Part model, mm, in its own coordinate system. Face numbers are marked on the shaded views. A direction names the side the tool comes from. Round coordinates to 2 decimals unless told otherwise and drop trailing zeros. Loops run counter-clockwise (first coordinate to the right, second up) from the corner with the lowest first, then second, coordinate; pieces in that order, holes last.
1) Band-saw the part on C-C, the plane y = 0. Write the cut outline in (x, z), then the cut area to 4 significant figures.
2) Drop flat-ended pins along their axis: P1, Ø2, axis at x = 14, y = -2, coming from the -Z side; P2, Ø3, axis at y = 1, z = -26.5, coming from the -X side; P3, Ø5, axis at x = 11.5, y = 0, coming from the -Z side; P4, Ø6.5, axis at y = -5, z = -11, coming from the +X side. Give the stop position or say it passes through.
3) Band-saw the part on A-A, the plane y = -5. Write the cut outline in (x, z).
4) 3-axis set-ups, long thin cutter, end or side, ignore diameter. For the marked faces 1, 2, 3 and 4: which of +Z, -Z, +X, -X, +Y, -Y reach the whole face in a straight line?
5) Band-saw the part on D-D, the plane z = -32.5. Write the cut outline in (x, y).
6) Probe line 1 (Y direction, x = 14.5, z = -17.3); line 2 (Y direction, x = -34, z = -17); line 3 (X direction, y = -2.5, z = -26.5). List the from-to ranges inside material, lowest first.
7) Band-saw the part on B-B, the plane x = 14.5. Write the cut outline in (y, z), then the cut area to 3 significant figures.
from build123d import *

# Parameters (mm, degrees)
PAD050_DEPTH    = 10
SKETCH087_R     = 2
POCKET033_DEPTH = 47.001
FILLET024_R     = 1


with BuildPart() as part:
    # Sketch086 → Pad050 (new body, symmetric)
    with BuildSketch(Plane.XZ):
        Polygon((-37, -18.5), (-37, -16), (-30, -16), (-30, -8), (10, -8), (10, -16), (17, -16), (17, -18.5), (10, -18.5), (10, -47), (-30, -47), (-30, -18.5), align=None)
    extrude(amount=PAD050_DEPTH, both=True)

    # Sketch087 → Pocket033 (cut, through all)
    with BuildSketch(Plane.XY):
        with Locations((14.5, 5)):
            Circle(SKETCH087_R)
        with Locations((14.5, -5)):
            Circle(SKETCH087_R)
        with Locations((-34.5, 5)):
            Circle(SKETCH087_R)
        with Locations((-34.5, -5)):
            Circle(SKETCH087_R)
    extrude(amount=-POCKET033_DEPTH, mode=Mode.SUBTRACT)

    # Fillet024
    fillet024_edges = [part.edges().sort_by_distance(p)[0] for p in [
        (17, -10, -17.25),
        (17, 10, -17.25),
        (-37, -10, -17.25),
        (-37, 10, -17.25),
    ]]
    fillet(fillet024_edges, radius=FILLET024_R)


solid = part.part
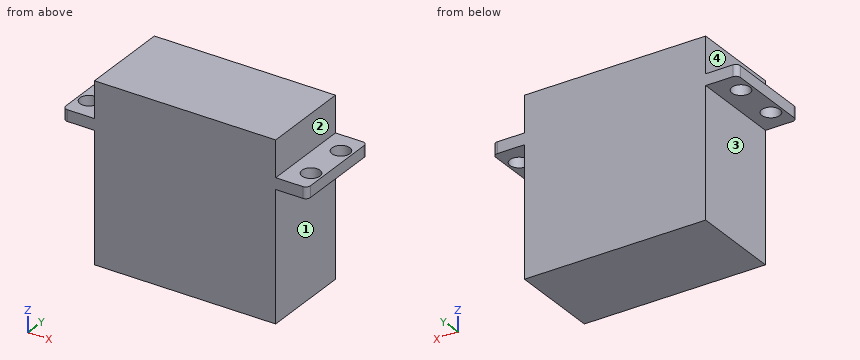
Reported:
1. outline: (-37, -18.5) - (-30, -18.5) - (-30, -47) - (10, -47) - (10, -18.5) - (17, -18.5) - (17, -16) - (10, -16) - (10, -8) - (-30, -8) - (-30, -16) - (-37, -16) - close
1. area: 1,595 mm2
2. P1: stops at z = -18.5
2. P2: stops at x = -30
2. P3: stops at z = -47
2. P4: stops at x = 10
3. outline: (-37, -18.5) - (-36.5, -18.5) - (-36.5, -16) - (-37, -16) - close; (-32.5, -18.5) - (-30, -18.5) - (-30, -47) - (10, -47) - (10, -18.5) - (12.5, -18.5) - (12.5, -16) - (10, -16) - (10, -8) - (-30, -8) - (-30, -16) - (-32.5, -16) - close; (16.5, -18.5) - (17, -18.5) - (17, -16) - (16.5, -16) - close
4. face 1: -Z, +X, +Y, -Y
4. face 2: +Z, +X, +Y, -Y
4. face 3: -Z, -X, +Y, -Y
4. face 4: +Z, -X, +Y, -Y
5. outline: (-30, -10) - (10, -10) - (10, 10) - (-30, 10) - close
6. line 1: y = -10 to -7, -3 to 3, 7 to 10
6. line 2: y = -10 to -6.94, -3.06 to 3.06, 6.94 to 10
6. line 3: x = -30 to 10
7. outline: (-10, -18.5) - (-7, -18.5) - (-7, -16) - (-10, -16) - close; (-3, -18.5) - (3, -18.5) - (3, -16) - (-3, -16) - close; (7, -18.5) - (10, -18.5) - (10, -16) - (7, -16) - close
7. area: 30.0 mm2
